Can you work these out from the drawing? Everything is in mm from the part's minimum corner. Round coordinates to 2 decimals unless told otherwise and drop trailing zeros. Loops run counter-clockwise (first coordinate to the right, second up) from the corner with the lowest first, then second, coordinate; pieces in that order, holes last. Notation, with made-up numbers: (78.5, -4) - (116.5, -4) arc R24 cw to (116.5, 10) - close; hole circle Ø10 at (0.25, -30). An arc over 180 degrees is marked (long way). Put each result on its own line as item: value. Start each with the question number.
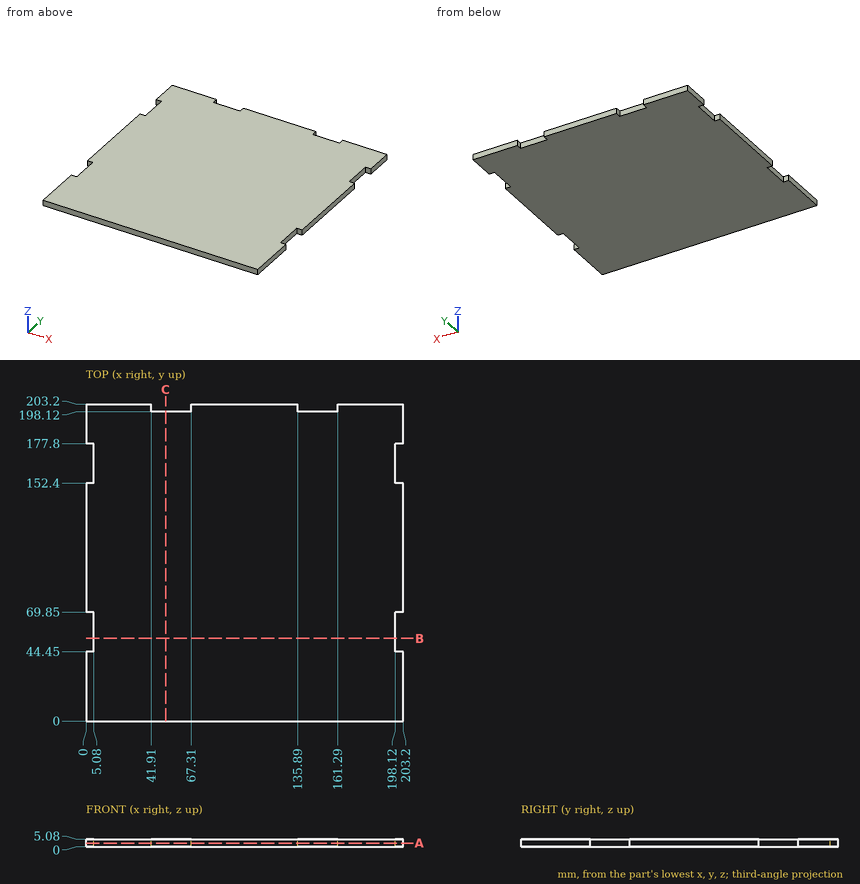
Item 1: I need wall thicknesses on line 1 (Y direction, x = 58.5, z = 2.95); line 2 (X direction, y = 175, z = 1.3). Which ranges of each line are inside material? Lowest first, please. Write a range as from..to.
Item 2: Suppose I cut it at B-B, the plane y = 53. List the corners of the cut face in (x, z) for me.
Item 3: Suppose I cut it at C-C, the plane x = 51. List the corners of the cut face in (y, z) for me.
Item 4: Will these pins go through, and if not, where does the flat tip stop? P1, Ø8, axis at x = 54, y = 51.5, coming from the -Z side; P2, Ø1, axis at y = 171.5, z = 1, coming from the +X side.
Item 5: Suppose I cut it at A-A, the plane z = 2.45. List the corners of the cut face in (x, y) for me, then the cut area to 3 significant figures.
Numbers:
1. line 1: 0..198.12
1. line 2: 5.08..198.12
2. outline: (5.08, 0) - (198.12, 0) - (198.12, 5.08) - (5.08, 5.08) - close
3. outline: (0, 0) - (198.12, 0) - (198.12, 5.08) - (0, 5.08) - close
4. P1: z = 0
4. P2: x = 198.12
5. outline: (0, 0) - (203.2, 0) - (203.2, 44.45) - (198.12, 44.45) - (198.12, 69.85) - (203.2, 69.85) - (203.2, 152.4) - (198.12, 152.4) - (198.12, 177.8) - (203.2, 177.8) - (203.2, 203.2) - (161.29, 203.2) - (161.29, 198.12) - (135.89, 198.12) - (135.89, 203.2) - (67.31, 203.2) - (67.31, 198.12) - (41.91, 198.12) - (41.91, 203.2) - (0, 203.2) - (0, 177.8) - (5.08, 177.8) - (5.08, 152.4) - (0, 152.4) - (0, 69.85) - (5.08, 69.85) - (5.08, 44.45) - (0, 44.45) - close
5. area: 40,500 mm^2
